Geometry check sheet. Reference: drawing and pictorial views, mm from the part's lowest x, y, z. A direction names the side the tool comes from. Round coordinates to 2 decimals unless told otherwise and drop trailing zeros. Write each loop counter-clockwise with the first axis right and the second up, starting at its lowest first coordinate (ties: lowest second). Pieces come first, ordered by that corner, then holes. Notation, with made-up numbers: (-38, 40.25) - (4, 40.25) arc R10 ccw to (4, 46.25) - close; hole circle Ø11 at (46.25, 8.25). An arc over 180 degrees is marked (long way). Return JSON: item names as keys, results as strings.
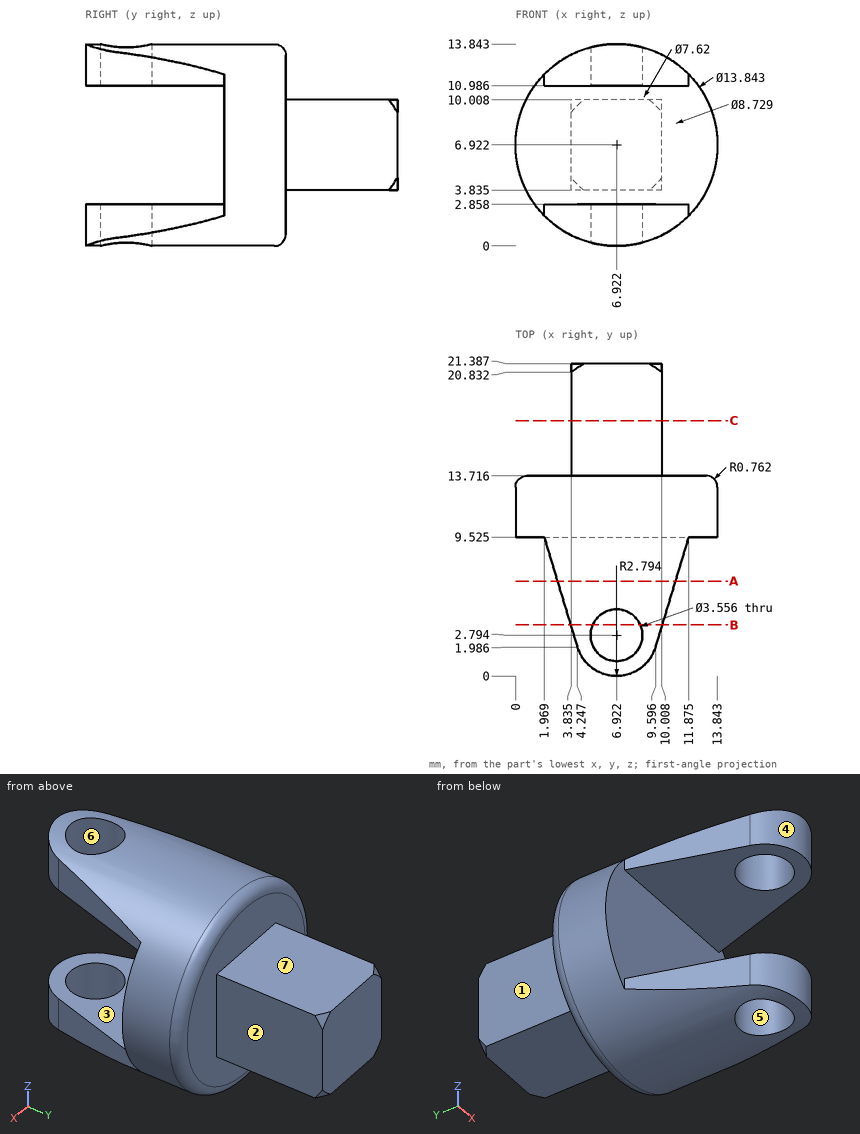
(1) Access from +Z, -Z, +X, -X, +Y, -Y to the whole of each face (thin tool, end or side, straight path). Record for the marked faces 1, 2 and 3.
Response values:
{"face 1": "+Z, -Z, -X, +Y", "face 2": "+Z, -Z, +X, +Y", "face 3": "+X, -X, -Y"}
(2) Section check C-C, the plane y = 17.5. Enter the section's corners in (x, z) (1 decimal).
Response values:
{"outline": "(3.8, 3.8) - (10, 3.8) - (10, 10) - (3.8, 10) - close"}
(3) Material ranges on line 1 along Y through (x, z) = (4.75, 3.25) (1 decimal); line 2 along Y through (x, z) = (5, 2) (1 decimal); line 3 along Z through (x, y) = (4.25, 14.75) (1 decimal), recorded low to high. Write a range as [from, to].
Response values:
{"line 1": "y = [9.5, 13.7]", "line 2": "y = [0.8, 13.7]", "line 3": "z = [3.8, 10]"}
(4) Section check B-B, the plane y = 3.5. Give the number of separate pieces and of enclosed holes in the cut face, plus the area to 3 significant figures.
Response values:
{"separate pieces": "4", "enclosed holes": "0", "area": "14.5 mm^2"}
(5) Section check A-A, the plane y = 6.5. Enter the section's corners in (x, z) (1 decimal).
Response values:
{"outline": "(2.9, 1.3) arc R6.9 ccw to (11, 1.3) - (11, 2.9) - (2.9, 2.9) - close; (2.9, 11) - (11, 11) - (11, 12.5) arc R6.9 ccw to (2.9, 12.5) - close"}
(6) Gauge pin test, flat ends, axial feed: pin 1 (1.9 mm diameter, centred on x = 6, y = 17.5, fed in from -Z) (1 decimal); pin 2 (2 mm diameter, centred on y = 10, z = 12, fed in from -X); pin 3 (3 mm diameter, centred on x = 7.5, y = 18, fed in from +Z). Record the tip position at first contact, or that the pin passes through.
Response values:
{"pin 1": "stops at z = 3.8", "pin 2": "stops at x = 1.33", "pin 3": "stops at z = 10.01"}
(7) Release check for a two-part mould opening along Y. For the marked faces 4, 5, 6 and 7 record: pulls with the +Y half, pulls with the -Y half, needs draft (parallel to the pull), parting line crosses it, or undercut.
Response values:
{"face 4": "pulls with the -Y half", "face 5": "undercut", "face 6": "undercut", "face 7": "needs draft"}
